Here's how the part is built. I have some questions about the finished solid (model axes, mm). A direction names the side the tool comes from. Give positions to 0.01 mm unless a question says otherwise; leave off trailing zeros. Loops run counter-clockwise (first coordinate to the right, second up) from the corner with the lowest first, then second, coordinate; pieces in that order, holes last. Notation, with made-up numbers: (75.5, 71.25) - (110.5, 71.25) arc R22 ccw to (110.5, 100.25) - close; hole circle Ø2 at (-7, -21). An arc over 180 degrees is marked (long way). Use a Markdown table: item, result.
from build123d import *

# Parameters (mm, degrees)
F0_R     = 5
F1_DEPTH = 27
F2_R     = 4
F3_DEPTH = 25
F4_R     = 1.75
F5_DEPTH = 25
F7_DEPTH = 6
F8_R     = 1
F9_DEPTH = 25


with BuildPart() as f1:
    # F0 (on Front) → F1 (new body)
    with BuildSketch(Plane.XZ):
        Circle(F0_R)
    extrude(amount=F1_DEPTH)

    # F2 (on face) → F3 (cut)
    with BuildSketch(Plane.XZ.offset(27)):
        Circle(F2_R)
    extrude(amount=-F3_DEPTH, mode=Mode.SUBTRACT)

    # F4 (on face) → F5 (cut)
    with BuildSketch(Plane(origin=(0, 0, 0), x_dir=(-1, 0, 0), z_dir=(0, 1, 0))):
        Circle(F4_R)
    extrude(amount=-F5_DEPTH, mode=Mode.SUBTRACT)

    # F6 (on face) → F7 (join)
    with BuildSketch(Plane(origin=(0, 0, 0), x_dir=(-1, 0, 0), z_dir=(0, 1, 0))):
        with BuildLine():
            Line((-11, -2), (-4.582575695, -2))
            ThreePointArc((-4.582575695, -2), (-5, 0), (-4.582575695, 2))
            Line((-4.582575695, 2), (-11, 2))
            Line((-11, 2), (-11, -2))
        make_face()
    extrude(amount=-F7_DEPTH)

    # F8 (on face) → F9 (cut)
    with BuildSketch(Plane(origin=(0, 0, -2), x_dir=(1, 0, 0), z_dir=(0, 0, -1))):
        with Locations((7.6, 3)):
            Circle(F8_R)
    extrude(amount=-F9_DEPTH, mode=Mode.SUBTRACT)


solid = f1.part
(1) Suppose I cut it at C-C on z = 1.25. Write out the boundary of the cut face in (x, y).
A:
| item | result |
|---|---|
| outline | (-4.84, -27) - (-3.8, -27) - (-3.8, -2) - (-1.22, -2) - (-1.22, 0) - (-4.84, 0) - close; (1.22, -2) - (3.8, -2) - (3.8, -27) - (4.84, -27) - (4.84, -6) - (11, -6) - (11, 0) - (1.22, 0) - close; hole circle Ø2 at (7.6, -3) |
(2) On a 3-axis mill with a long thin cutter (end or side, diameter ignored), from which of +Z, -Z, +X, -X, +Y, -Y can I reach the whole of each face in a straight line? I mean faces 1 (the face through (9, -2, -2)), 2 (the face through (6.863, -3.676, -0.028)), 3 (the face through (2, -2, -1)). Say none if no direction works.
A:
| item | result |
|---|---|
| face 1 | -Z, +X, +Y, -Y |
| face 2 | +Z, -Z |
| face 3 | -Y |
(3) Will these pins go through, and if not, where does the flat tip stop? pin 1 (3 mm diameter, centred on x = 6.5, z = 1, fed in from -Y); pin 2 (2 mm diameter, centred on x = 7, z = 2.5, fed in from +Y); pin 3 (3 mm diameter, centred on x = 0, z = 0, fed in from -Y); pin 4 (3 mm diameter, centred on x = 7.6, y = -3, fed in from +Z).
A:
| item | result |
|---|---|
| pin 1 | y = -6 |
| pin 2 | y = 0 |
| pin 3 | through |
| pin 4 | z = 2 |
(4) We'd pull the mould along X, two halves only. Please class faces 4 (the face through (7.7, -1.6, 2)), 5 (the face through (-1.617, -0.986, -0.67)), 6 (the face through (-5, -13, 0)): pulls with the +X half, pulls with the -X half, needs draft (parallel to the pull), parting line crosses it, or undercut.
A:
| item | result |
|---|---|
| face 4 | needs draft |
| face 5 | undercut |
| face 6 | parting line crosses it |
(5) Suppose I cut it at D-D on x = 0. Write out the boundary of the cut face in (y, z), plus the area to 3 significant figures.
A:
| item | result |
|---|---|
| outline | (-27, -5) - (0, -5) - (0, -1.75) - (-2, -1.75) - (-2, -4) - (-27, -4) - close; (-27, 4) - (-2, 4) - (-2, 1.75) - (0, 1.75) - (0, 5) - (-27, 5) - close |
| area | 63.0 mm2 |
(6) Suppose I cut it at B-B on x = 7.6. Write out the boundary of the cut face in (y, z).
A:
| item | result |
|---|---|
| outline | (-6, -2) - (-4, -2) - (-4, 2) - (-6, 2) - close; (-2, -2) - (0, -2) - (0, 2) - (-2, 2) - close |
(7) Suppose I cut it at A-A on y = -3. Write out the boundary of the cut face in (x, z).
A:
| item | result |
|---|---|
| outline | (4.58, -2) - (6.6, -2) - (6.6, 2) - (4.58, 2) arc R5 ccw (long way) to start; (8.6, -2) - (11, -2) - (11, 2) - (8.6, 2) - close; hole circle Ø8 at (0, 0) |
(8) If I drill on line 1 (X direction, y = -3, z = -0.05); line 2 (Z direction, x = 0, y = -20.25); line 3 (Y direction, x = 7.6, z = -0.5), over which ranges is the centre line in solid material (lowest first)?
A:
| item | result |
|---|---|
| line 1 | -5 to -4, 4 to 6.6, 8.6 to 11 |
| line 2 | -5 to -4, 4 to 5 |
| line 3 | -6 to -4, -2 to 0 |
